Read the model definition and answer for the solid it produces. Units are mm, in the model's axes. Face numbers are marked on the shaded views. A direction names the side the tool comes from. Coordinates: 2 decimals unless noted, no trailing zeros. Order: outer loops, then holes, each group sorted by start corner. A loop starts at its lowest first (then second) coordinate and runs counter-clockwise, first axis right, second up.
```python
from build123d import *

# Parameters (mm, degrees)
SKETCH2_W                = 240
SKETCH2_H                = 30
BOSS_EXTRUDE1_DEPTH      = 5
BOSS_EXTRUDE2_DEPTH      = 6
BOSS_EXTRUDE3_DEPTH      = 2
BOSS_EXTRUDE3_DEPTH_BACK = 9
SKETCH4_W                = 26
SKETCH4_H                = 2
SKETCH5_W                = 26
SKETCH5_H                = 1.998827679
BOSS_EXTRUDE4_DEPTH      = 2
SKETCH6_W                = 26
SKETCH6_H                = 2
BOSS_EXTRUDE5_DEPTH      = 2
SKETCH8_W                = 76.2
SKETCH8_H                = 2
CUT_EXTRUDE1_DEPTH       = 6
SKETCH9_W                = 10
SKETCH9_H                = 1.3
CUT_EXTRUDE2_DEPTH       = 40
FILLET1_R                = 0.5


with BuildPart() as part:
    # Sketch2 → Boss-Extrude1 (new body)
    with BuildSketch(Plane(origin=(0, 0, 0), x_dir=(1, 0, 0), z_dir=(0, 1, 0))):
        with Locations((120, -15)):
            Rectangle(SKETCH2_W, SKETCH2_H)
    extrude(amount=BOSS_EXTRUDE1_DEPTH)

    # Sketch3 → Boss-Extrude2 (add)
    with BuildSketch(Plane(origin=(0, 5, 0), x_dir=(1, 0, 0), z_dir=(0, 1, 0))):
        Polygon((90, 0), (85.819507893, 0), (85.819507893, -30), (141.819507893, -30), (141.819507893, 0), (138.819507893, 0), (138.819507893, -26), (117.819507893, -26), (117.819507893, 0), (111, 0), (111, -26), (90, -26), align=None)
    extrude(amount=BOSS_EXTRUDE2_DEPTH)

    # Sketch4 → Boss-Extrude3 (add, two sides: drawn at the far end of the back side and taken through both)
    with BuildSketch(Plane.ZY.offset(-111).offset(-BOSS_EXTRUDE3_DEPTH_BACK)):
        with Locations((13, 10)):
            Rectangle(SKETCH4_W, SKETCH4_H)
    extrude(amount=BOSS_EXTRUDE3_DEPTH + BOSS_EXTRUDE3_DEPTH_BACK)

    # Sketch5 → Boss-Extrude4 (add)
    with BuildSketch(Plane(origin=(90, 0, 0), x_dir=(0, 0, -1), z_dir=(1, 0, 0))):
        with Locations((-13, 10.00058616)):
            Rectangle(SKETCH5_W, SKETCH5_H)
    extrude(amount=BOSS_EXTRUDE4_DEPTH)

    # Sketch6 → Boss-Extrude5 (add)
    with BuildSketch(Plane.ZY.offset(-138.819507893)):
        with Locations((13, 10)):
            Rectangle(SKETCH6_W, SKETCH6_H)
    extrude(amount=BOSS_EXTRUDE5_DEPTH)

    # Sketch8 → Cut-Extrude1 (cut)
    with BuildSketch(Plane(origin=(0, 5, 0), x_dir=(1, 0, 0), z_dir=(0, 1, 0))):
        with Locations((192.9, -25)):
            Rectangle(SKETCH8_W, SKETCH8_H)
        with Locations((192.9, -5)):
            Rectangle(SKETCH8_W, SKETCH8_H)
    extrude(amount=-CUT_EXTRUDE1_DEPTH, mode=Mode.SUBTRACT)

    # Sketch9 → Cut-Extrude2 (cut)
    with BuildSketch(Plane.ZY):
        with Locations((14.996078434, 0.65)):
            Rectangle(SKETCH9_W, SKETCH9_H)
        Polygon((21.2, 1.3), (21.2, 3.5), (15, 3.5), (8.8, 3.5), (8.8, 1.3), align=None)
    extrude(amount=-CUT_EXTRUDE2_DEPTH, mode=Mode.SUBTRACT)

    # Fillet1
    fillet1_edges = [part.edges().sort_by_distance(p)[0] for p in [
        (192.9, 0, 26),
        (42.909753947, 5, 30),
        (192.9, 5, 4),
        (192.9, 5, 6),
        (192.9, 5, 24),
        (240, 5, 15),
        (190.909753947, 5, 30),
        (100.5, 5, 0),
        (128.319507893, 5, 0),
        (190.909753947, 5, 0),
        (42.909753947, 5, 0),
        (85.819507893, 8, 0),
        (85.819507893, 8, 30),
        (141.819507893, 8, 30),
        (141.819507893, 8, 0),
        (113.819507893, 11, 30),
        (139.319507893, 11, 0),
        (114.5, 11, 0),
        (88.909753947, 11, 0),
        (111, 7, 0),
        (117.819507893, 7, 0),
        (118.909753947, 9, 0),
        (120, 10, 0),
        (120, 0, 0),
        (110, 9, 0),
        (109, 10, 0),
        (120, 0, 30),
        (90, 7.000586161, 0),
        (91, 9.001172321, 0),
        (92, 10.000586161, 0),
        (138.819507893, 7, 0),
        (0, 2.5, 0),
        (137.819507893, 9, 0),
        (240, 2.5, 0),
        (136.819507893, 10, 0),
        (240, 2.5, 30),
        (0, 2.5, 30),
    ]]
    fillet(fillet1_edges, radius=FILLET1_R)


solid = part.part
```
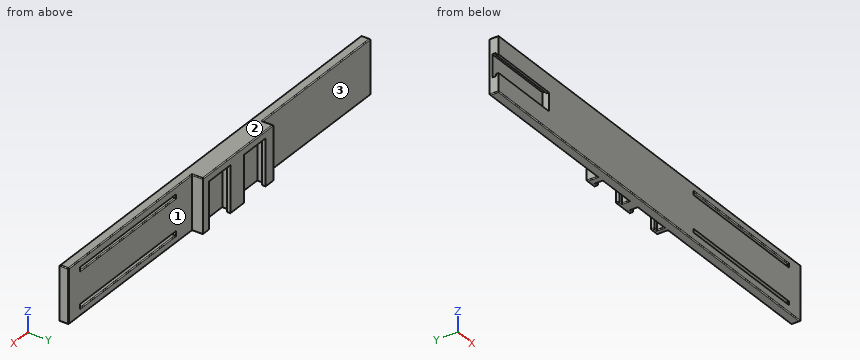
1) Flat-ended cylindrical pins translate along their axes: pin 1 Ø2 at (y, z) = (7.5, 12.5) entering from -X; pin 2 Ø4.5 at (y, z) = (8, 10) entering from +X; pin 3 Ø1.8 at (x, y) = (99, 7) entering from -Z. Find the tip coordinate at first contact, or state that the pin passes through.
A:
pin 1: stops at x = 85.82
pin 2: stops at x = 141.82
pin 3: stops at z = 26
2) A cutting plane is placed at B-B, the plane z = 12.5. Determine the outline of the cut face in (x, y).
A:
outline: (0, 3.5) - (40, 3.5) - (40, 0) - (240, 0) - (240, 4.5) arc R0.5 ccw to (239.5, 5) - (141.82, 5) - (141.82, 11) - (136.82, 11) - (136.82, 9) - (138.82, 9) - (138.82, 5) - (117.82, 5) - (117.82, 9) - (120, 9) - (120, 11) - (109, 11) - (109, 9) - (111, 9) - (111, 5) - (90, 5) - (90, 9) - (92, 9) - (92, 11) - (85.82, 11) - (85.82, 5) - (0, 5) - close
3) Which of the six approach directions +Z, -Z, +X, -X, +Y, -Y give full straight-line access (tool end or side, diameter ignored) to the marked faces 1, 2 and 3?
A:
face 1: +Z, -Z, +X, +Y
face 2: +Z, +X, -X, +Y, -Y
face 3: +Z, -Z, -X, +Y
4) A cutting plane is placed at C-C, the plane x = 64. Determine the outline of the cut face in (y, z), and give its area (3 significant figures).
A:
outline: (0, 0.5) arc R0.5 ccw to (0.5, 0) - (4.5, 0) arc R0.5 ccw to (5, 0.5) - (5, 29.5) arc R0.5 ccw to (4.5, 30) - (0.5, 30) arc R0.5 ccw to (0, 29.5) - close
area: 150 mm2
5) A cutting plane is placed at A-A, the plane y = 7.25. Determine the outline of the cut face in (x, z), and give its area (3 significant figures).
A:
outline: (85.82, 0.5) arc R0.5 ccw to (86.32, 0) - (89.5, 0) arc R0.5 ccw to (90, 0.5) - (90, 26) - (111, 26) - (111, 0.5) arc R0.5 ccw to (111.5, 0) - (117.32, 0) arc R0.5 ccw to (117.82, 0.5) - (117.82, 26) - (138.82, 26) - (138.82, 0.5) arc R0.5 ccw to (139.32, 0) - (141.32, 0) arc R0.5 ccw to (141.82, 0.5) - (141.82, 29.5) arc R0.5 ccw to (141.32, 30) - (86.32, 30) arc R0.5 ccw to (85.82, 29.5) - close
area: 588 mm2
6) A cutting plane is placed at D-D, the plane x = 25.5. Determine the outline of the cut face in (y, z), and give its area (3 significant figures).
A:
outline: (0, 0.5) arc R0.5 ccw to (0.5, 0) - (4.5, 0) arc R0.5 ccw to (5, 0.5) - (5, 29.5) arc R0.5 ccw to (4.5, 30) - (0.5, 30) arc R0.5 ccw to (0, 29.5) - (0, 20) - (1.3, 20) - (1.3, 21.2) - (3.5, 21.2) - (3.5, 8.8) - (1.3, 8.8) - (1.3, 10) - (0, 10) - close
area: 110 mm2
7) Straight lines are drawn through the part: line 1 (X direction, y = 8, z = 22.75); line 2 (X direction, y = 9.5, z = 15.5); line 3 (Z direction, x = 222, y = 1). For each, find the intervals that lie inside material, in ascending order.
A:
line 1: x = 85.82 to 90, 111 to 117.82, 138.82 to 141.82
line 2: x = 85.82 to 92, 109 to 120, 136.82 to 141.82
line 3: z = 0 to 4, 6 to 24, 26 to 30
